Autodesk Inventor part; units mm, degrees
ref_plane "YZ Plane" through (0, 0, 0) normal (1, 0, 0) x (0, 1, 0)
ref_plane "XZ Plane" through (0, 0, 0) normal (0, 1, 0) x (-1, 0, 0)
ref_plane "XY Plane" through (0, 0, 0) normal (0, 0, 1) x (1, 0, 0)
sketch "Sketch1" plane through (0, 0, 0) normal (0, 0, 1) x (1, 0, 0)
  line L0 (0, 0) -> (60, 0)
  line L1 (60, 0) -> (60, 70)
  line L2 (60, 70) -> (0, 70)
  line L3 (0, 70) -> (0, 0)
  dimension "d0" = 60
  dimension "d1" = 70
extrude "Extrusion1" add sketch "Sketch1" along normal blind 10
sketch "Sketch2" plane through (0, 0, 10) normal (0, 0, 1) x (1, 0, 0)
  line L0 (0, 60) -> (60, 60) construction
  line L1 (60, 0) -> (60, 70) construction
  line L2 (0, 60) -> (60, 0) construction
  line L3 (0, 0) -> (60, 0) construction
  line L4 (60, 60) -> (0, 0) construction
  arc A0 (0, 0) -> (0, 60) centre (-23.1222, 30) ccw construction
  arc A1 (60, 60) -> (60, 0) centre (83.1222, 30) ccw construction
  line L5 (60, 70) -> (0, 70) construction
  line L6 (30, 70) -> (30, 0) construction
  line L7 (17.3619, 30) -> (14.7544, 30) construction
  line L8 (42.6381, 30) -> (45.2456, 30) construction
  line L9 (0, 60) -> (60, 60)
  circle A2 centre (30, 10.6788) radius 10.6788
  line L10 (19.3212, 10.6788) -> (19.3212, 25.6788)
  line L11 (6.8778, 53.1222) -> (0, 60)
  line L12 (40.6788, 10.6788) -> (40.6788, 25.6788)
  line L13 (60, 60) -> (53.1222, 53.1222)
  line L14 (6.8778, 53.1222) -> (19.3212, 25.6788)
  line L15 (53.1222, 53.1222) -> (40.6788, 25.6788)
  line L16 (0, 70) -> (0, 0)
  line L17 (0, 60) -> (0, 70)
  line L18 (0, 70) -> (60, 70)
  line L19 (60, 70) -> (60, 60)
  line L20 (40.6788, 25.6788) -> (19.3212, 25.6788)
  line L21 (53.1222, 53.1222) -> (6.8778, 53.1222)
  line L22 (6.8778, 53.1222) -> (0, 60)
  line L23 (53.1222, 53.1222) -> (60, 60)
  line L24 (0, 70) -> (0, 0)
  line L25 (0, 60) -> (0, 70)
  line L26 (0, 70) -> (60, 70)
  line L27 (60, 60) -> (60, 70)
  dimension "d4" = 10
extrude "Extrusion2" add sketch "Sketch2" along normal blind 10
sketch "Sketch3" plane through (60, 0, 0) normal (1, 0, 0) x (0, 0, -1)
  line L0 (-10, 60) -> (-20, 60)
  line L1 (-10, 60) -> (-10, 70)
  line L2 (0, 70) -> (-20, 70)
  line L3 (0, 0) -> (-10, 0)
  line L4 (-10, 0) -> (0, 0)
  line L5 (-10, 60) -> (-10, 0)
  line L6 (-10, 0) -> (-10, 60)
  line L7 (0, 0) -> (0, 70)
  line L8 (-10, 0) -> (0, 0)
  line L9 (0, 0) -> (0, 70)
  line L10 (0, 70) -> (-10, 70)
extrude "Extrusion3" cut sketch "Sketch3" against normal through all
sketch "Sketch4" plane through (0, 0, 20) normal (0, 0, 1) x (1, 0, 0)
  arc A0 (19.3212, 10.6788) -> (40.6788, 10.6788) centre (30, 10.6788) ccw construction
  line L0 (30, 10.6788) -> (30, 0) construction
  line L1 (60, 70) -> (0, 70) construction
  line L2 (30, 70) -> (30, 10.6788) construction
  circle A1 centre (30, 10.6788) radius 7.9826 construction
  circle A2 centre (30, 10.6788) radius 7.9826
  point P0 (0, 0)
extrude "Extrusion4" cut sketch "Sketch4" against normal blind 10
properties part number "Wheel Holder"
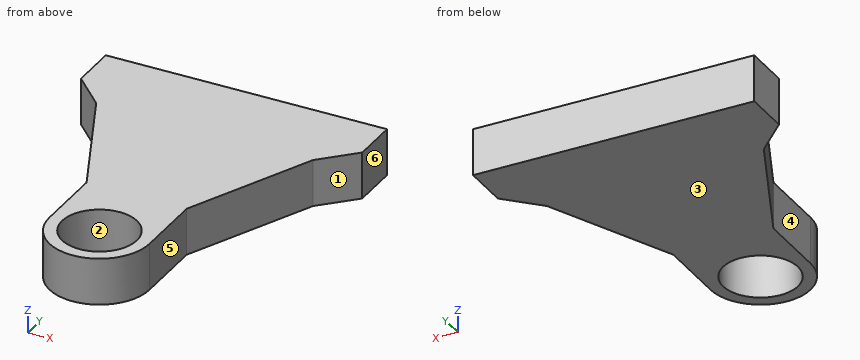
For this review, take the finished solid that the model builds, in its own axes (mm). Face numbers are marked on the shaded views. A direction names the side the tool comes from. Give positions to 0.01 mm unless a question says otherwise; leave off trailing zeros. Write each loop counter-clockwise with the first axis right and the second up, starting at its lowest first coordinate (ties: lowest second). Pieces come first, ordered by that corner, then holes. Notation, with made-up numbers: M 81,48 L 89,48 A17 cw 89,80 Z; hole C 64.5,-29 d8. An arc over 180 degrees is marked long. Answer as a JSON object with one key per item and string values. Group by question number.
Item 1: Tool access review of the marked faces 4, 5 and 6: name each direction out of +Z, -Z, +X, -X, +Y, -Y from which nothing blocks a thin tool from reaching the whole face with its end or side.
Item 2: Consider section B-B on z = 12. Write out the cut boundary in (x, y).
Item 3: Consider section D-D on y = 22. Write out the cut boundary in (x, z).
Item 4: Consider section C-C on y = 5. Write out the cut boundary in (x, z), plus the area to 3 significant figures.
Item 5: For pin 1 Ø5 at (x, z) = (53, 15.5) entering from -Y; pin 2 Ø1.5 at (x, z) = (25, 16) entering from -Y; pin 3 Ø5 at (y, z) = (9, 17.5) entering from -X, all flat-tipped, find the tip position at first contact; note any pin that passes through.
Item 6: Consider section A-A on x = 30. Write out the cut boundary in (y, z), plus the area to 3 significant figures.
Item 7: For probe 1 along X at (y, z) = (10.5, 15.75); probe 2 along Y at (x, z) = (30, 15); probe 3 along X at (y, z) = (8, 13.5), list the stretches that pass through material, from the lowest coordinate up. Write a range as [from, to].
Item 8: Draft analysis for pull direction X (two halves, no side actions). For the marked faces 1, 2 and 3, state which applies: +X half, -X half, draft (parallel to the pull), parting line (faces both ways), or undercut.
Check result:
{
 "1": {"face 4": "+Z, -Z, -X, -Y", "face 5": "+Z, -Z, +X, -Y", "face 6": "+Z, -Z, +X, +Y, -Y"},
 "2": {"outline": "M 0,60 L 6.88,53.12 L 19.32,25.68 L 19.32,10.68 A10.68 ccw 40.68,10.68 L 40.68,25.68 L 53.12,53.12 L 60,60 L 60,70 L 0,70 Z; hole C 30,10.68 d15.97"},
 "3": {"outline": "M 19.32,10 L 40.68,10 L 40.68,20 L 19.32,20 Z"},
 "4": {"outline": "M 20.96,10 L 24.39,10 L 24.39,20 L 20.96,20 Z; M 35.61,10 L 39.04,10 L 39.04,20 L 35.61,20 Z", "area": "68.7 mm^2"},
 "5": {"pin 1": "stops at y = 47.34", "pin 2": "stops at y = 0.88", "pin 3": "stops at x = 19.32"},
 "6": {"outline": "M 0,10 L 2.7,10 L 2.7,20 L 0,20 Z; M 18.66,10 L 70,10 L 70,20 L 18.66,20 Z", "area": "540 mm^2"},
 "7": {"probe 1": "x = [19.32, 22.02], [37.98, 40.68]", "probe 2": "y = [0, 2.7], [18.66, 70]", "probe 3": "x = [19.66, 22.48], [37.52, 40.34]"},
 "8": {"face 1": "+X half", "face 2": "undercut", "face 3": "draft"}
}
